```python
from build123d import *

# Parameters (mm, degrees)
AXLE_BASE_SKETCH_R        = 15.5
AXLE_DEPTH                = 93.5
GUARD_BASE_R              = 25
GUARD_DEPTH               = 5
INNER_AXLE_HOLE_BASE_R    = 8.5
INNER_AXLE_HOLE_DEPTH     = 99.5
BEND_ROOM_BASE_W          = 1.5
BEND_ROOM_BASE_H          = 50
BEND_ROOM_1_DEPTH         = 45
BEND_ROOM_2_COUNT         = 2
BEND_ROOM_2_ANGLE         = 90
EASY_REMOVAL_CHAMFER_SIZE = 4


with BuildPart() as part:
    # Axle base sketch → Axle (new body)
    with BuildSketch(Plane.XY):
        Circle(AXLE_BASE_SKETCH_R)
    extrude(amount=AXLE_DEPTH)

    # Guard base → Guard (add)
    with BuildSketch(Plane(origin=(0, 0, 0), x_dir=(-1, 0, 0), z_dir=(0, 0, -1))):
        Circle(GUARD_BASE_R)
    extrude(amount=GUARD_DEPTH)

    # Inner axle hole base → Inner axle hole (cut, through all)
    with BuildSketch(Plane.XY.offset(93.5)):
        Circle(INNER_AXLE_HOLE_BASE_R)
    extrude(amount=-INNER_AXLE_HOLE_DEPTH, mode=Mode.SUBTRACT)

    # Mate ring base → Mate rings (revolve)
    with BuildSketch(Plane(origin=(0, 0, 0), x_dir=(1, 0, 0), z_dir=(0, 1, 0))):
        Polygon((15.5, -93.5), (16.25, -92.75), (16.25, -92), (15.5, -91.25), align=None)
        Polygon((15.5, -87.75), (16.25, -87), (16.25, -86.25), (15.5, -85.5), align=None)
    revolve(axis=Axis((0, 0, 0), (0, 0, -1)))

    # Bend room base → Bend room 1 (cut)
    with BuildSketch(Plane.XY.offset(93.5)):
        Rectangle(BEND_ROOM_BASE_W, BEND_ROOM_BASE_H)
    bend_room_1 = extrude(amount=-BEND_ROOM_1_DEPTH, mode=Mode.SUBTRACT)

    # Bend room 2: Bend room 1 ×2 about axis
    bend_room_2_axis = Axis((0, 0, 0), (0, 0, -1))
    for i in range(1, BEND_ROOM_2_COUNT):
        add(bend_room_1.rotate(bend_room_2_axis, i * BEND_ROOM_2_ANGLE / (BEND_ROOM_2_COUNT - 1)), mode=Mode.SUBTRACT)

    # Easy removal chamfer
    easy_removal_chamfer_edges = [part.edges().sort_by_distance(p)[0] for p in [
        (25, 0, 0),
    ]]
    chamfer(easy_removal_chamfer_edges, length=EASY_REMOVAL_CHAMFER_SIZE)


solid = part.part
```
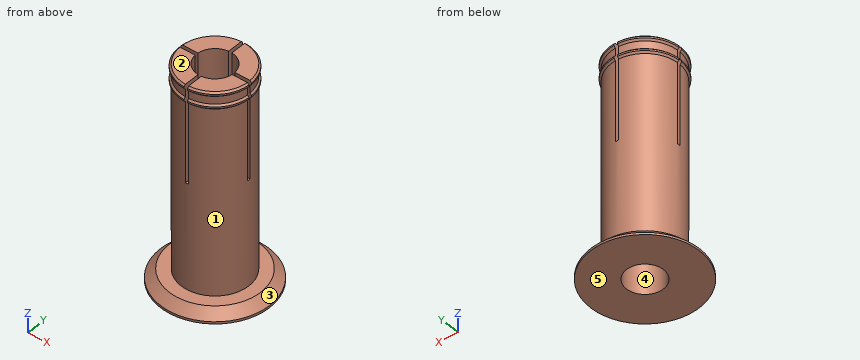
The listing builds one solid part. Answer for the finished solid, in the listing's coordinates (mm). Face numbers are marked on the shaded views. A direction names the side the tool comes from. Round coordinates to 2 decimals unless told otherwise and drop trailing zeros. Write each loop counter-clockwise with the first axis right and the second up, starting at its lowest first coordinate (ties: lowest second). Pieces come first, ordered by that corner, then holes. Notation, with made-up numbers: (34.5, -35.75) -> (70.5, -35.75) arc R16 cw to (70.5, -26.75) -> close; hole circle Ø3 at (40.5, 16.25). An arc over 180 degrees is marked (long way). Write item = value, one per line.
1) Which of the six approach directions +Z, -Z, +X, -X, +Y, -Y give full straight-line access (tool end or side, diameter ignored) to the marked faces 1 and 2?
Check values:
face_1 = none
face_2 = +Z, +X, -X, +Y, -Y
2) Section A-A on z = 71 is taken. Write down the section's boundary in (x, y), plus the area to 3 significant figures.
Check values:
outline = (-15.48, -0.75) arc R15.5 ccw to (-0.75, -15.48) -> (-0.75, -8.47) arc R8.5 cw to (-8.47, -0.75) -> close; (-15.48, 0.75) -> (-8.47, 0.75) arc R8.5 cw to (-0.75, 8.47) -> (-0.75, 15.48) arc R15.5 ccw to start; (0.75, -15.48) arc R15.5 ccw to (15.48, -0.75) -> (8.47, -0.75) arc R8.5 cw to (0.75, -8.47) -> close; (0.75, 8.47) arc R8.5 cw to (8.47, 0.75) -> (15.48, 0.75) arc R15.5 ccw to (0.75, 15.48) -> close
area = 486 mm²
3) Section B-B on z = 24.5 is taken. Write down the section's boundary in (x, y).
Check values:
outline = circle Ø31 at (0, 0); hole circle Ø17 at (0, 0)
4) Straight lines are drawn through the part: line 1 along Y through (x, z) = (0, 42); line 2 along Z through (x, y) = (-18.5, -7.5); line 3 along Y through (x, z) = (2, 40). For each, find the intervals that lie inside material, in ascending order. Write a range as [from, to].
Check values:
line_1 = [-15.5, -8.5], [8.5, 15.5]
line_2 = [-5, 0]
line_3 = [-15.37, -8.26], [8.26, 15.37]
5) Given pin 1 (1.2 mm diameter, centred on x = 0.5, y = 13, fed in from +Z); pin 2 (1.5 mm diameter, centred on x = 12.5, z = 5, fed in from +Y); pin 3 (6 mm diameter, centred on x = -11, z = 63.5, fed in from +Y); pin 4 (13.5 mm diameter, centred on x = 0, y = 0, fed in from -Z), each flat-ended and moving along its own axis, determine where each tip first touches the part or whether it passes through.
Check values:
pin_1 = 93.5
pin_2 = 10.11
pin_3 = 13.28
pin_4 = through
6) For a pull along Y with two mould halves and no side action, classify the marked faces 3, 4 and 5 as released by +Y, released by -Y, zero draft, split by the parting line, or undercut.
Check values:
face_3 = split by the parting line
face_4 = undercut
face_5 = zero draft
